Design review of the part built by this model. Coordinates are the model's own, in mm. A direction names the side the tool comes from. Round coordinates to 2 decimals unless told otherwise and drop trailing zeros. Loops run counter-clockwise (first coordinate to the right, second up) from the corner with the lowest first, then second, coordinate; pieces in that order, holes last. Notation, with made-up numbers: (2.5, 28) - (7.5, 28) arc R36 ccw to (7.5, 65) - close; hole circle Ø11 at (-35.75, 5.5). An arc over 180 degrees is marked (long way). One line per question, with ' | ' between items. Start each with the question number.
from build123d import *

# Parameters (mm, degrees)
CROQUIS1_W                        = 57
CROQUIS1_H                        = 24.959470006
CROQUIS1_W_2                      = 43
CROQUIS1_H_2                      = 22
MAIN_DEPTH                        = 28
CORTE_CAJA_REACH                  = 56.604
CROQUIS2_W                        = 27.955905163
CROQUIS2_H                        = 20.987971864
CROQUIS3_W                        = 32
CROQUIS3_H                        = 24.959470006
SALIENTE_EXTRUIR2_DEPTH           = 2.25
REDONDEO_LATERALES_R              = 3
CROQUIS7_R                        = 1.3
TALADROS_BASE_DEPTH               = 11
CAJEADO_CABLE_DEPTH               = 10
CAJEADO_REDONDEO_R                = 2
SOPORTE_EN_ANGULO_DEPTH           = 24.959470007
CAJA_PARA_SOPORTE_DEPTH           = 11
CROQUIS12_R                       = 1.3
TALADROS_CAJA_SOPORTE_DEPTH       = 13.959470007
CROQUIS15_W                       = 60.00042655
CROQUIS15_H                       = 27.426571923
RECORTE_CAJA_DEPTH                = 24.959470007
CHAFLAN_SUPERIOR_SOPORTE_DEPTH    = 24.959470007
REDONDEO_ARISTAS_SOPORTE_R        = 3
REDONDEO_SOPORTE_R                = 14
CROQUIS17_W                       = 6.155207263
CROQUIS17_H                       = 26
CAJA_TORNILLOS_SOPORTE_DEPTH      = 8
REDONDEO_CAJA_TORNILLOS_SOPORTE_R = 3


with BuildPart() as part:
    # Croquis1 → Main (new body)
    with BuildSketch(Plane(origin=(0, 0, 0), x_dir=(1, 0, 0), z_dir=(0, 1, 0))):
        with Locations((11.181999645, 13.428246359)):
            Rectangle(CROQUIS1_W, CROQUIS1_H)
        with Locations((10.844499645, 13.338562849)):
            Rectangle(CROQUIS1_W_2, CROQUIS1_H_2, mode=Mode.SUBTRACT)
    extrude(amount=MAIN_DEPTH)

    # Corte Caja: up to this face of the body (flat: up to its plane)
    corte_caja_end = Plane(part.part.faces().sort_by_distance((11.181999645, 14, -25.907981362))[0])
    # Croquis2 → Corte Caja (cut, up to the picked face)
    with BuildSketch(Plane.XY.offset(-0.948511356), mode=Mode.PRIVATE) as corte_caja_sk1:
        with Locations((28.659952227, 20.493985932)):
            Rectangle(CROQUIS2_W, CROQUIS2_H)
    corte_caja_tool1 = split(extrude(corte_caja_sk1.sketch, amount=-CORTE_CAJA_REACH, mode=Mode.PRIVATE), bisect_by=corte_caja_end, keep=Keep.BOTH, mode=Mode.PRIVATE)
    add(corte_caja_tool1.solids().sort_by(Axis((28.659952, 20.493986, -0.948511), (0, 0, -1)))[0], mode=Mode.SUBTRACT)

    # Croquis3 → Saliente-Extruir2 (add)
    with BuildSketch(Plane(origin=(0, 28, 0), x_dir=(1, 0, 0), z_dir=(0, 1, 0))):
        with Locations((-1.318000355, 13.428246359)):
            Rectangle(CROQUIS3_W, CROQUIS3_H)
    extrude(amount=SALIENTE_EXTRUIR2_DEPTH)

    # Redondeo Laterales
    redondeo_laterales_edges = [part.edges().sort_by_distance(p)[0] for p in [
        (39.681999645, 5, -25.907981362),
        (39.681999645, 5, -0.948511356),
    ]]
    fillet(redondeo_laterales_edges, radius=REDONDEO_LATERALES_R)

    # Croquis7 → Taladros Base (cut)
    with BuildSketch(Plane.XZ):
        with Locations(Location((-13.155500355, -8.338562849, 0), (0, 0, 270))):
            Circle(CROQUIS7_R)
        with Locations(Location((-13.155500355, -18.338562849, 0), (0, 0, 270))):
            Circle(CROQUIS7_R)
        with Locations(Location((34.844499645, -8.338562849, 0), (0, 0, 270))):
            Circle(CROQUIS7_R)
        with Locations(Location((34.844499645, -18.338562849, 0), (0, 0, 270))):
            Circle(CROQUIS7_R)
    extrude(amount=-TALADROS_BASE_DEPTH, mode=Mode.SUBTRACT)

    # Croquis8 → Cajeado cable (cut)
    with BuildSketch(Plane.XZ):
        Polygon((-10.655500355, -17.197519433), (-10.655500355, -9.671098091), (-13.962983419, -11.385752006), (-13.962983419, -15.059503242), align=None)
    extrude(amount=-CAJEADO_CABLE_DEPTH, mode=Mode.SUBTRACT)

    # Cajeado Redondeo
    cajeado_redondeo_edges = [part.edges().sort_by_distance(p)[0] for p in [
        (-13.962983419, 5, -11.385752006),
        (-10.655500355, 5, -9.671098091),
        (-10.655500355, 5, -17.197519433),
        (-13.962983419, 5, -15.059503242),
    ]]
    fillet(cajeado_redondeo_edges, radius=CAJEADO_REDONDEO_R)

    # Croquis10 → Soporte en angulo (add)
    with BuildSketch(Plane.XY.offset(-0.948511356)):
        Polygon((-17.318000355, 30.25), (-17.318000355, 0), (-40.697936457, 0), (-44.719041018, 3.698501078), (-22.354269001, 32.502718411), (-18.018493057, 32.502718411), align=None)
    extrude(amount=-SOPORTE_EN_ANGULO_DEPTH)

    # Croquis11 → Caja para soporte (cut)
    with BuildSketch(Plane(origin=(0, 0, -25.907981362), x_dir=(-1, 0, 0), z_dir=(0, 0, -1))):
        with BuildLine():
            Line((41.509326916, 7.83238192), (25.563983103, 28.36883757))
            Line((25.563983103, 28.36883757), (21.614664709, 25.302425298))
            ThreePointArc((21.614664709, 25.302425298), (20.477989634, 23.307419605), (21.084921035, 21.092986898))
            Line((21.084921035, 21.092986898), (33.350570122, 5.295713321))
            ThreePointArc((33.350570122, 5.295713321), (35.345575815, 4.159038247), (37.560008522, 4.765969648))
            Line((37.560008522, 4.765969648), (41.509326916, 7.83238192))
        make_face()
    extrude(amount=-CAJA_PARA_SOPORTE_DEPTH, mode=Mode.SUBTRACT)

    # Croquis12 → Taladros caja soporte (cut)
    with BuildSketch(Plane(origin=(0, 0, -14.907981362), x_dir=(-1, 0, 0), z_dir=(0, 0, -1))):
        with Locations((27.011052418, 19.330608197)):
            Circle(CROQUIS12_R)
        with Locations((33.143876962, 11.431971409)):
            Circle(CROQUIS12_R)
    extrude(amount=-TALADROS_CAJA_SOPORTE_DEPTH, mode=Mode.SUBTRACT)

    # Croquis15 → Recorte Caja (cut)
    with BuildSketch(Plane.XY.offset(-0.948511356)):
        with Locations((11.033774869, 23.713285962)):
            Rectangle(CROQUIS15_W, CROQUIS15_H)
    extrude(amount=-RECORTE_CAJA_DEPTH, mode=Mode.SUBTRACT)

    # Croquis16 → Chaflan superior soporte (cut)
    with BuildSketch(Plane(origin=(0, 0, -25.907981362), x_dir=(-1, 0, 0), z_dir=(0, 0, -1))):
        Polygon((26.059899943, 33.268736427), (17.368016439, 26.520002701), (17.368016439, 33.268736427), align=None)
    extrude(amount=-CHAFLAN_SUPERIOR_SOPORTE_DEPTH, mode=Mode.SUBTRACT)

    # Redondeo aristas soporte
    redondeo_aristas_soporte_edges = [part.edges().sort_by_distance(p)[0] for p in [
        (-40.697936457, 0, -13.428246359),
        (-18.966438406, 27.761082869, -13.428246359),
    ]]
    fillet(redondeo_aristas_soporte_edges, radius=REDONDEO_ARISTAS_SOPORTE_R)

    # Redondeo soporte
    # the kernel refuses this fillet: 14 mm, written as the material it takes off along each edge
    with BuildSketch(Plane(origin=(-66.183926921, -23.946727682, -0.948511356), x_dir=(0.7898636788540391, -0.6132824543610909, 0), z_dir=(0.6132824543610909, 0.7898636788540392, 0))) as redondeo_soporte_piece_1:
        with BuildLine():
            CenterArc((REDONDEO_SOPORTE_R, REDONDEO_SOPORTE_R), REDONDEO_SOPORTE_R, 180, 90)
            Line((0, REDONDEO_SOPORTE_R), (0, 0))
            Line((0, 0), (REDONDEO_SOPORTE_R, 0))
        make_face()
    extrude(amount=104.799778712, mode=Mode.SUBTRACT)

    # Croquis17 → Caja tornillos soporte (cut)
    with BuildSketch(Plane(origin=(-29.691111601, 23.053392988, 0), x_dir=(0, 0, 1), z_dir=(-0.789863678854039, 0.6132824543610911, 0))):
        with Locations((-3.077603632, -6.270427893)):
            Rectangle(CROQUIS17_W, CROQUIS17_H)
    extrude(amount=-CAJA_TORNILLOS_SOPORTE_DEPTH, mode=Mode.SUBTRACT)

    # redondeo Caja tornillos soporte
    redondeo_caja_tornillos_soporte_edges = [part.edges().sort_by_distance(p)[0] for p in [
        (-35.190417485, 2.926122285, -4.227303989),
        (-19.245073672, 23.462577935, -4.227303989),
    ]]
    fillet(redondeo_caja_tornillos_soporte_edges, radius=REDONDEO_CAJA_TORNILLOS_SOPORTE_R)


solid = part.part
1. The part is to be moulded in two halves that separate along Z. For faces 1 (the face through (-20.482, 23.34, -20.485)), 2 (the face through (38.78, 5.07, -1.804)), 3 (the face through (-13.713, 5.07, -14.939)), say which applies: pulls with the +Z half, pulls with the -Z half, needs draft (parallel to the pull), parting line crosses it, or undercut.
2. To check wall thickness, follow line 1 along Z through (x, y) = (6.5, 3.5); line 2 along Y through (x, z) = (29.5, -1.75); line 3 along X through (y, z) = (3, -5.5). State the ranges of each line that lie inside material, in increasing order.
3. Clearance check with flat-ended pins moving along their axes: P1, Ø12, axis at x = 3.5, y = 11.5, coming from the +Z side; P2, Ø17, axis at x = -34.5, y = 18.5, coming from the -Z side; P3, Ø9.5, axis at x = -33.5, y = 15, coming from the +Z side; P4, Ø3.5, axis at x = -13.16, z = -18.34, coming from the +Y side. State where each tip first meets the part, or that it passes through.
4. Take a section at A-A, the plane z = -20.75. Give the boundary of the cut face in (x, y).
5. Machinability: for faces 4 (the face through (-20.482, 23.34, -4.629)), 5 (the face through (11, 5, -24.339)), 6 (the face through (10, 10, -2)), which of the approach directions +Z, -Z, +X, -X, +Y, -Y give a long, thin tool a straight path to every point of the face, cutting with its end or side? Answer none if there is none.
6. Take a section at B-B, the plane x = 3. Give the boundary of the cut face in (y, z), then the cut area to 3 significant figures.
Answer list:
1) face 1: needs draft | face 2: pulls with the +Z half | face 3: undercut
2) line 1: z = -25.91 to -24.34, -2.34 to -0.95 | line 2: y = 0 to 10 | line 3: x = -40.62 to -10.66, 32.34 to 39.68
3) P1: stops at z = -0.95 | P2: stops at z = -14.91 | P3: stops at z = -6.16 | P4: stops at y = 10
4) outline: (-44.72, 3.7) - (-41.56, 0.79) arc R3 ccw to (-39.53, 0) - (-10.66, 0) - (-10.66, 10) - (-18.97, 10) - (-18.97, 26.29) arc R3 ccw to (-20.13, 28.66) - (-23.38, 31.19) - (-25.56, 28.37) - (-21.61, 25.3) arc R3 cw to (-21.08, 21.09) - (-33.35, 5.3) arc R3 cw to (-37.56, 4.77) - (-41.51, 7.83) - close; (32.34, 0) - (39.68, 0) - (39.68, 10) - (32.34, 10) - close
5) face 4: +Z, -X | face 5: +Y, -Y | face 6: +Z, -Z, +X, +Y
6) outline: (0, -25.91) - (10, -25.91) - (10, -24.34) - (0, -24.34) - close; (0, -2.34) - (10, -2.34) - (10, -0.95) - (0, -0.95) - close | area: 29.6 mm²
